Verification items for the finished model (mm, model axes). Face numbers are marked on the shaded views. A direction names the side the tool comes from. Give positions to 0.01 mm unless a question says otherwise; leave off trailing zeros. Write each loop counter-clockwise with the first axis right and the second up, starting at its lowest first coordinate (ties: lowest second). Pieces come first, ordered by that corner, then holes.
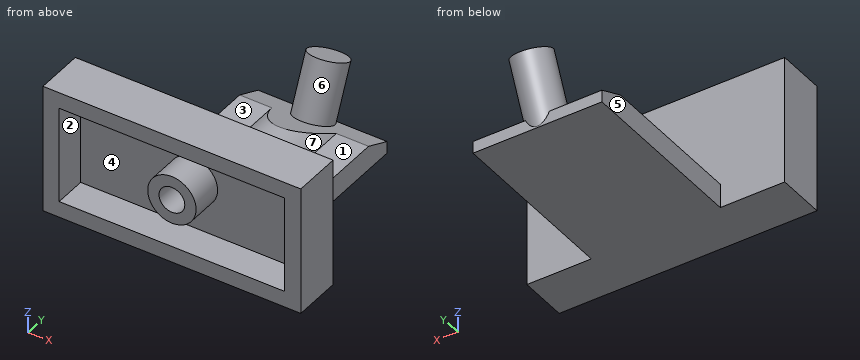
from build123d import *

# Parameters (mm, degrees)
SKETCH1_W                       = 16
SKETCH1_H                       = 8
BOSS_EXTRUDE1_DEPTH             = 3
SHELL1_T                        = -1
SKETCH2_R                       = 1.5
SKETCH2_R_2                     = 0.8
BOSS_EXTRUDE2_DEPTH             = 2
BOSS_EXTRUDE3_DEPTH             = 11
CUT_EXTRUDE1_DEPTH              = 13
BOSS_EXTRUDE4_REACH             = 8.299
SKETCH5_R                       = 1.2
BOSS_EXTRUDE4_DIRECTION_2_DEPTH = 3.5


with BuildPart() as part:
    # Sketch1 → Boss-Extrude1 (new body)
    with BuildSketch(Plane(origin=(0, 0, 0), x_dir=(1, 0, 0), z_dir=(0, 1, 0))):
        Rectangle(SKETCH1_W, SKETCH1_H)
    extrude(amount=BOSS_EXTRUDE1_DEPTH)

    # Shell1
    shell1_openings = [part.faces().sort_by_distance(p)[0] for p in [
        (0, 0, 0),
    ]]
    offset(amount=SHELL1_T, openings=shell1_openings, kind=Kind.INTERSECTION)

    # Sketch2 → Boss-Extrude2 (add)
    with BuildSketch(Plane.XZ.offset(-2)):
        Circle(SKETCH2_R)
        Circle(SKETCH2_R_2, mode=Mode.SUBTRACT)
    extrude(amount=BOSS_EXTRUDE2_DEPTH)

    # Sketch3 → Boss-Extrude3 (add)
    with BuildSketch(Plane(origin=(0, 3, 0), x_dir=(1, 0, 0), z_dir=(0, 1, 0))):
        with BuildLine():
            Line((-4, 4), (4, 4))
            Line((4, 4), (4, 2.5))
            Line((4, 2.5), (2, 2.5))
            ThreePointArc((2, 2.5), (0, 1.5), (-2, 2.5))
            Line((-2, 2.5), (-4, 2.5))
            Line((-4, 2.5), (-4, 4))
        make_face()
    extrude(amount=BOSS_EXTRUDE3_DEPTH)

    # Sketch4 → Cut-Extrude1 (cut, through all)
    with BuildSketch(Plane(origin=(4, 0, 0), x_dir=(0, 0, -1), z_dir=(1, 0, 0))):
        Polygon((3.25, 14), (1.5, 14), (1.5, 10), align=None)
    extrude(amount=-CUT_EXTRUDE1_DEPTH, mode=Mode.SUBTRACT)

    # Sketch5 → Boss-Extrude4 (add, up to next)
    with BuildSketch(Plane(origin=(0, 1.055737705, 2.413114754), x_dir=(1, 0, 0), z_dir=(0, 0.400818834, 0.916157335)), mode=Mode.PRIVATE) as boss_extrude4_sk1:
        with Locations((0, 13.193279121)):
            Circle(SKETCH5_R)
    boss_extrude4_tool1 = extrude(boss_extrude4_sk1.sketch, amount=-BOSS_EXTRUDE4_REACH, mode=Mode.PRIVATE) - part.part
    add(boss_extrude4_tool1.solids().sort_by_distance((0, 13.142857, -2.875))[0])

    # Sketch5 → Boss-Extrude4 direction 2 (add)
    with BuildSketch(Plane(origin=(0, 1.055737705, 2.413114754), x_dir=(1, 0, 0), z_dir=(0, 0.400818834, 0.916157335))):
        with Locations((0, 13.193279121)):
            Circle(SKETCH5_R)
    extrude(amount=BOSS_EXTRUDE4_DIRECTION_2_DEPTH)


solid = part.part
Item 1: Set-up check for the marked faces 1, 2 and 3: record each of +Z, -Z, +X, -X, +Y, -Y from which the full face is reachable in a straight line by a thin tool's end or side.
Answer key:
face 1: +Z, +X, +Y
face 2: -Y
face 3: +Z, -X, +Y
Item 2: Depth check by flat-ended pin: pin 1 (1.7 mm diameter, centred on y = 9.5, z = -3.5, fed in from +X); pin 2 (1 mm diameter, centred on y = 4.5, z = 0.5, fed in from +X); pin 3 (1.6 mm diameter, centred on y = 6.5, z = -3.5, fed in from -X); pin 4 (0.6 mm diameter, centred on x = -3.5, y = 8.5, fed in from +Z). Enter the tip coordinate at first touch or a pass-through.
Answer key:
pin 1: stops at x = 4
pin 2: passes through
pin 3: stops at x = -4
pin 4: stops at z = -2.5
Item 3: Release check for a two-part mould opening along Y. For the marked faces 4, 5, 6 and 7 record: released by +Y, released by -Y, zero draft, split by the parting line, or undercut.
Answer key:
face 4: released by -Y
face 5: zero draft
face 6: undercut
face 7: undercut
Item 4: Scan lines: line 1 along Z through (x, y) = (0, 0.65); line 2 along X through (y, z) = (1.5, -1.25); line 3 along Y through (x, z) = (6.5, -2.5). Record each from-to range of solid material in increasing order.
Answer key:
line 1: z = -4 to -3, -1.5 to -0.8, 0.8 to 1.5, 3 to 4
line 2: x = -8 to -7, -0.83 to 0.83, 7 to 8
line 3: y = 2 to 3
Item 5: Sectioned sample at D-D on x = -5. Record the cut outline in (y, z).
Answer key:
outline: (0, -4) - (3, -4) - (3, 4) - (0, 4) - (0, 3) - (2, 3) - (2, -3) - (0, -3) - close
Item 6: Sectioned sample at C-C on z = 3.75. Record the cut outline in (x, y).
Answer key:
outline: (-8, 0) - (8, 0) - (8, 3) - (-8, 3) - close
Item 7: Sectioned sample at A-A on y = 1. Record the cut outline in (x, z).
Answer key:
outline: (-8, -4) - (8, -4) - (8, 4) - (-8, 4) - close; circle Ø3 at (0, 0); hole (-7, -3) - (7, -3) - (7, 3) - (-7, 3) - close; hole circle Ø1.6 at (0, 0)
Item 8: Sectioned sample at B-B on x = 3.75. Record the cut outline in (y, z).
Answer key:
outline: (0, -4) - (14, -4) - (14, -3.25) - (12.29, -2.5) - (3, -2.5) - (3, 4) - (0, 4) - (0, 3) - (2, 3) - (2, -3) - (0, -3) - close
